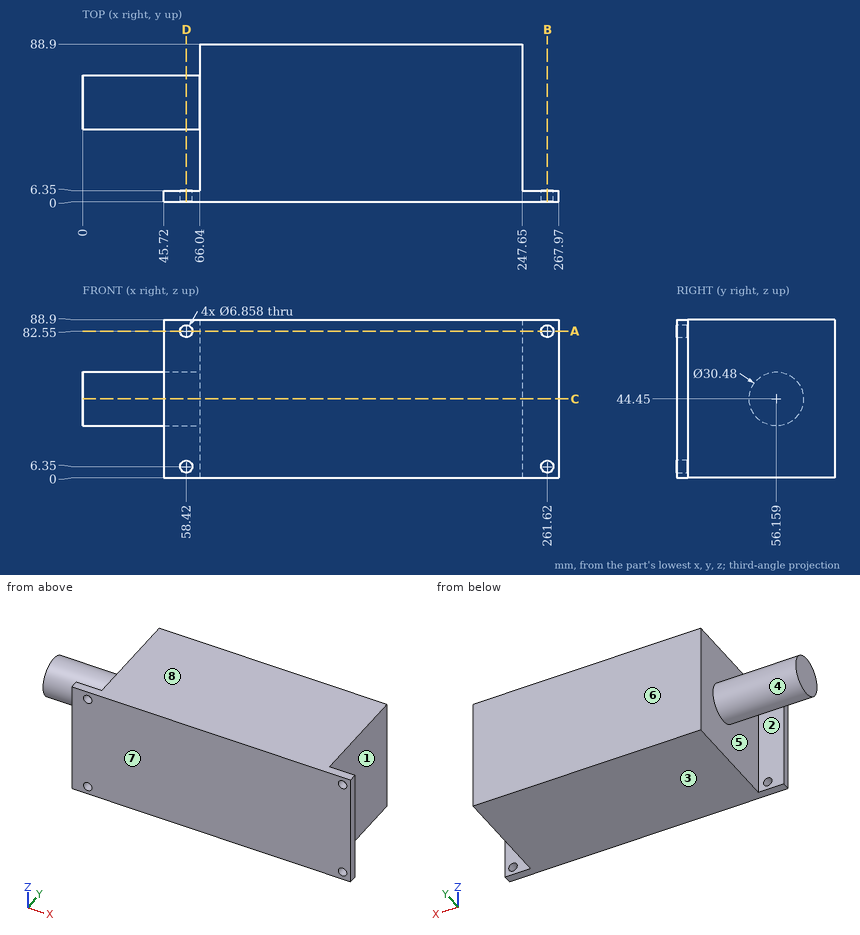
Part print with two shaded views. Sizes in mm from the minimum x, y, z corner. A direction names the side the tool comes from. Coordinates: 2 decimals unless noted, no trailing zeros. Write each loop counter-clockwise with the first axis right and the second up, starting at its lowest first coordinate (ties: lowest second). Pieces come first, ordered by that corner, then holes.
(1) Cut at D-D on x = 58.42. List the corners of the cut face in (y, z), and give its area (3 significant figures).
(2) Cut at A-A on z = 82.55. List the corners of the cut face in (x, y), and give its area (3 significant figures).
(3) Cut at B-B on x = 261.62. List the corners of the cut face in (y, z).
(4) Pin check, flat tips, straight feed: pin 1 Ø22.5 at (x, z) = (261.5, 56) entering from +Y; pin 2 Ø25 at (y, z) = (38, 23) entering from +X; pin 3 Ø1.5 at (x, z) = (67.5, 11.5) entering from -Y; pin 4 Ø3 at (x, y) = (62.5, 44) entering from -Z. Stop position of each tip, or through.
(5) Mould opens along Y. For the marked faces 5, 6, 7 and 8 say: pulls with the +Y half, pulls with the -Y half, needs draft (parallel to the pull), parting line crosses it, or undercut.
(6) 3-axis set-ups, long thin cutter, end or side, ignore diameter. For the marked faces 1, 2, 3 and 4: which of +Z, -Z, +X, -X, +Y, -Y reach the whole face in a straight line?
(7) Drill centre lines: line 1 (X direction, y = 2.5, z = 6.35); line 2 (Z direction, x = 261, y = 1); line 3 (Z direction, x = 58, y = 3). Where is each one in solid material? Low to high.
(8) Cut at C-C on z = 44.45. List the corners of the cut face in (x, y), and give its area (3 significant figures).
Working result:
1. outline: (0, 0) - (6.35, 0) - (6.35, 2.92) - (0, 2.92) - close; (0, 9.78) - (6.35, 9.78) - (6.35, 79.12) - (0, 79.12) - close; (0, 85.98) - (6.35, 85.98) - (6.35, 88.9) - (0, 88.9) - close; circle Ø30.48 at (56.16, 44.45)
1. area: 1,210 mm2
2. outline: (45.72, 0) - (54.99, 0) - (54.99, 6.35) - (45.72, 6.35) - close; (61.85, 0) - (258.19, 0) - (258.19, 6.35) - (247.65, 6.35) - (247.65, 88.9) - (66.04, 88.9) - (66.04, 6.35) - (61.85, 6.35) - close; (265.05, 0) - (267.97, 0) - (267.97, 6.35) - (265.05, 6.35) - close
2. area: 16,300 mm2
3. outline: (0, 0) - (6.35, 0) - (6.35, 2.92) - (0, 2.92) - close; (0, 9.78) - (6.35, 9.78) - (6.35, 79.12) - (0, 79.12) - close; (0, 85.98) - (6.35, 85.98) - (6.35, 88.9) - (0, 88.9) - close
4. pin 1: stops at y = 6.35
4. pin 2: stops at x = 247.65
4. pin 3: stops at y = 0
4. pin 4: stops at z = 33.56
5. face 5: undercut
5. face 6: pulls with the +Y half
5. face 7: pulls with the -Y half
5. face 8: needs draft
6. face 1: +Z, -Z, +X, +Y
6. face 2: +Z, -Z, -X
6. face 3: -Z, +X, -X, +Y, -Y
6. face 4: -X
7. line 1: x = 45.72 to 54.99, 61.85 to 258.19, 265.05 to 267.97
7. line 2: z = 0 to 2.98, 9.72 to 79.18, 85.92 to 88.9
7. line 3: z = 0 to 2.95, 9.75 to 79.15, 85.95 to 88.9
8. outline: (0, 40.92) - (66.04, 40.92) - (66.04, 6.35) - (45.72, 6.35) - (45.72, 0) - (267.97, 0) - (267.97, 6.35) - (247.65, 6.35) - (247.65, 88.9) - (66.04, 88.9) - (66.04, 71.4) - (0, 71.4) - close
8. area: 18,400 mm2
